Part model, mm, in its own coordinate system. A direction names the side the tool comes from. Round coordinates to 2 decimals unless told otherwise and drop trailing zeros. Order: outer loops, then holes, each group sorted by start corner. A loop starts at its lowest first (then second) coordinate and runs counter-clockwise, first axis right, second up. Notation, with made-up numbers: (-24.5, 80.5) -> (26.5, 80.5) arc R17 cw to (26.5, 87.5) -> close; hole circle Ø2 at (-6.75, 14.5). An arc over 180 degrees is marked (long way). Use CSV: the item, a comma, the result in double quotes.
```python
from build123d import *

# Parameters (mm, degrees)
F0_R         = 8
F0_R_2       = 6.5
F1_DEPTH     = 11.5
F0_R_3       = 12.5
F2_DEPTH     = 4.25
F3_S5_R      = 8
F3_T6_DEPTH  = 19
F3_S11_R     = 8
F3_T12_DEPTH = 19
F0_R_4       = 5.5
F5_DEPTH     = 7.5
F6_SIZE      = 0.99999


# Not quite as in the source:
# - a fillet or chamfer that OpenCascade refuses, or shapes differently, is made with other operations: its cross-section is extruded or revolved along the edge and cut away or added
# - two fillets or chamfers of one size are made in one step
# - a fillet or chamfer is up to 0.001 mm smaller than in the source, because OpenCascade refuses the exact size


with BuildPart() as f1:
    # F0 (on Top) → F1 (new body, symmetric)
    with BuildSketch(Plane.XY):
        Circle(F0_R)
        Circle(F0_R_2, mode=Mode.SUBTRACT)
    extrude(amount=F1_DEPTH, both=True)

    # F0 (on Top) → F2 (join, symmetric)
    with BuildSketch(Plane.XY):
        Circle(F0_R_3)
        Circle(F0_R, mode=Mode.SUBTRACT)
    extrude(amount=F2_DEPTH, both=True)

    # F3: chamfer of 5 x 4 on 2 edges, made by hand


with BuildPart() as f3_tool2:
    # F3_s3 → F3_t4 (revolve)
    with BuildSketch(Plane.XZ):
        Polygon((12.5, 0.25), (7.5, 4.25), (12.5, 4.25), align=None)
    revolve(axis=Axis((0, 0, 4.25), (0, 0, 1)))

    # F3_s5 → F3_t6 (cut, symmetric)
    with BuildSketch(Plane.XY.offset(2.2)):
        Circle(F3_S5_R)
    extrude(amount=F3_T6_DEPTH, both=True, mode=Mode.SUBTRACT)


with BuildPart() as f1_1:
    add(f1.part)

    # F3_t1: cut F3_tool2
    add(f3_tool2.part, mode=Mode.SUBTRACT)


with BuildPart() as f3_tool8:
    # F3_s9 → F3_t10 (revolve)
    with BuildSketch(Plane.XZ):
        Polygon((7.5, -4.25), (12.5, -0.25), (12.5, -4.25), align=None)
    revolve(axis=Axis((0, 0, -4.25), (0, 0, 1)))

    # F3_s11 → F3_t12 (cut, symmetric)
    with BuildSketch(Plane.XY.offset(-2.2)):
        Circle(F3_S11_R)
    extrude(amount=F3_T12_DEPTH, both=True, mode=Mode.SUBTRACT)


with BuildPart() as f1_2:
    add(f1_1.part)

    # F3_t7: cut F3_tool8
    add(f3_tool8.part, mode=Mode.SUBTRACT)

    # F0 (on Top) → F5 (join, symmetric)
    with BuildSketch(Plane.XY):
        Circle(F0_R_2)
        Circle(F0_R_4, mode=Mode.SUBTRACT)
    extrude(amount=F5_DEPTH, both=True)

    # F6 (size 1 in the source; OpenCascade refuses exactly that, so slightly less here)
    f6_edges = [f1_2.edges().sort_by_distance(p)[0] for p in [
        (-5.5, 0, 7.5),
    ]]
    chamfer(f6_edges, length=F6_SIZE)


solid = f1_2.part
```
(1) Pull direction X, two halves, no side cores. Call faces 1 (the face through (-8.211, 0.361, 3.675)), 2 (the face through (0, 7, -11.5)), 3 (the face through (-5.158, -3.955, -9.528)): released by +X, released by -X, zero draft, split by the parting line, or undercut.
Reply:
face 1,"split by the parting line"
face 2,"zero draft"
face 3,"undercut"
(2) Which spindle directions (+Z, -Z, +X, -X, +Y, -Y) get a long thin tool onto all of the face, cutting with end or side? Do faces 4 (the face through (-5.158, -3.955, 9.472)), 5 (the face through (-5, 3, -7.5)), 6 (the face through (-1.19, -5.37, -0.6)). Say none if no direction does.
Reply:
face 4,"+Z"
face 5,"-Z"
face 6,"+Z, -Z"
(3) Cut at C-C, the plane z = -8.5. Give the cut face in (x, y), then the cut area to 3 significant figures.
Reply:
outline,"circle Ø16 at (0, 0); hole circle Ø13 at (0, 0)"
area,"68.3 mm2"
(4) Probe probe 1 along Y at (x, z) = (0, 9.5); probe 2 along Y at (x, z) = (0, -4.25); probe 3 along X at (y, z) = (-2.25, -2). List the from-to ranges inside material, lowest first. Write a range as [from, to].
Reply:
probe 1,"[-8, -6.5], [6.5, 8]"
probe 2,"[-8, -5.5], [5.5, 8]"
probe 3,"[-10.06, -5.02], [5.02, 10.06]"
(5) Drop flat-ended pins along their axis: P1, Ø12, axis at y = 6.5, z = -8, coming from the -X side; P2, Ø3, axis at x = 7.5, y = 9.5, coming from the +Z side; P3, Ø2, axis at x = -2, z = 0.5, coming from the +Y side. Give the stop position or say it passes through.
Reply:
P1,"x = -8.8"
P2,"z = 1.77"
P3,"y = 12.46"
